from build123d import *

# Parameters (mm, degrees)
F0_W      = 114.494712
F0_H      = 62.637055
F1_DEPTH  = 25.4
F2_R      = 10.795138
F2_R_2    = 10.841205
F2_R_3    = 10.79514
F3_DEPTH  = 116.84
F5_DEPTH  = 42.926
F6_W      = 51.59115
F6_H      = 62.667213
F7_DEPTH  = 11.176
F8_R      = 10.847006
F9_DEPTH  = 65.532
F10_W     = 18.654421
F10_H     = 20.111804
F10_W_2   = 18.65442
F10_H_2   = 17.488524
F11_DEPTH = 45.212


with BuildPart() as f1:
    # F0 (on Front) → F1 (new body)
    with BuildSketch(Plane.XZ):
        with Locations((-4.824847, 5.261216)):
            Rectangle(F0_W, F0_H)
    extrude(amount=F1_DEPTH)

    # F2 (on Front) → F3 (cut)
    with BuildSketch(Plane.XZ):
        with Locations((13.092266, 4.241542)):
            Circle(F2_R)
        with Locations((-28.568659, 5.406883)):
            Circle(F2_R_2)
        with Locations((-28.568659, 5.406883)):
            Circle(F2_R_3, mode=Mode.SUBTRACT)
        with Locations((-28.568659, 5.406883)):
            Circle(F2_R_3)
    extrude(amount=F3_DEPTH, mode=Mode.SUBTRACT)

    # F4 (on Front) → F5 (join)
    with BuildSketch(Plane.XZ):
        Polygon((-42.860791, -25.608312), (-42.860791, 36.285762), (-62.284995, 36.472697), (-62.284995, -26.409047), align=None)
    extrude(amount=F5_DEPTH)

    # F6 (on Front) → F7 (join)
    with BuildSketch(Plane.XZ):
        with Locations((-36.28869, 5.246557)):
            Rectangle(F6_W, F6_H)
    extrude(amount=-F7_DEPTH)

    # F8 (on Front) → F9 (cut)
    with BuildSketch(Plane.XZ):
        with Locations((-26.232786, 2.563626)):
            Circle(F8_R)
    extrude(amount=-F9_DEPTH, mode=Mode.SUBTRACT)

    # F10 (on Front) → F11 (join)
    with BuildSketch(Plane.XZ):
        with Locations((42.555411, -15.739673)):
            Rectangle(F10_W, F10_H)
        with Locations((42.55541, 27.835902)):
            Rectangle(F10_W_2, F10_H_2)
    extrude(amount=F11_DEPTH)


solid = f1.part
The listing builds one solid part. Answer for the finished solid, in the listing's coordinates (mm). A direction names the side the tool comes from. Give positions to 0.01 mm unless a question says otherwise; leave off trailing zeros. Loops run counter-clockwise (first coordinate to the right, second up) from the corner with the lowest first, then second, coordinate; pieces in that order, holes last. Notation, with made-up numbers: (-17, 86) - (22, 86) arc R18 cw to (22, 95) - close; hole circle Ø9 at (72, 12). An arc over 180 degrees is marked (long way). Use one line per item in the form item = value.
1. Section C-C on x = 39 is taken. Give the vertices of the cut face in (y, z).
Calculated:
outline = (-45.21, -25.8) - (-25.4, -25.8) - (-25.4, -26.06) - (0, -26.06) - (0, 36.58) - (-45.21, 36.58) - (-45.21, 19.09) - (-25.4, 19.09) - (-25.4, -5.68) - (-45.21, -5.68) - close
2. Section D-D on x = 17.5 is taken. Give the vertices of the cut face in (y, z), then the cut area to 3 significant figures.
Calculated:
outline = (-25.4, -26.06) - (0, -26.06) - (0, -5.61) - (-25.4, -5.61) - close; (-25.4, 14.1) - (0, 14.1) - (0, 36.58) - (-25.4, 36.58) - close
area = 1,090 mm^2
3. The mould has two halves that part along X. Classify faces 1 (the face through (-10.493, 6, 5)), 2 (the face through (42, -22, 36.58)), 3 (the face through (33.228, -35, -16)): pulls with the +X half, pulls with the -X half, needs draft (parallel to the pull), parting line crosses it, or undercut.
Calculated:
face_1 = pulls with the +X half
face_2 = needs draft
face_3 = undercut
4. Find the intervals of material crossed by line 1 along X through (y, z) = (-39, -6) (3 decimals); line 2 along Z through (x, y) = (35, -40.5); line 3 along Y through (x, z) = (42, -3), in increasing order. Write a range as [from, to].
Calculated:
line_1 = [-62.285, -42.861], [33.228, 51.883]
line_2 = [-25.8, -5.68], [19.09, 36.58]
line_3 = [-25.4, 0]
5. Section B-B on z = 7 is taken. Count the separate pieces of the cut face and the enclosed holes in it, then the cut area to 3 significant figures.
Calculated:
separate_pieces = 3
enclosed_holes = 0
area = 2,530 mm^2
6. Given pin 1 Ø5.5 at (y, z) = (-34, 17.5) entering from +X; pin 2 Ø25 at (x, z) = (13.09, 4.24) entering from -Y; pin 3 Ø10 at (y, z) = (-26, 6) entering from +X; pin 4 Ø21 at (x, z) = (-33, 10.5) entering from -Y, each flat-ended and moving along its own axis, determine where each tip first touches the part or whether it passes through.
Calculated:
pin_1 = 51.88
pin_2 = -25.4
pin_3 = 52.42
pin_4 = -42.93
7. Which of the six approach directions +Z, -Z, +X, -X, +Y, -Y give full straight-line access (tool end or side, diameter ignored) to faces 4 (the face through (-21, 0, -3)), 5 (the face through (42, -35, -5.684)), 6 (the face through (42, -35, -25.796))?
Calculated:
face_4 = +Y
face_5 = +X, -Y
face_6 = -Z, +X, -Y
8. Section A-A on y = -38.5 is taken. Give the vertices of the cut face in (x, z) (3 decimals), then the cut area to 3 significant figures.
Calculated:
outline = (-62.285, -26.409) - (-42.861, -25.608) - (-42.861, 36.286) - (-62.285, 36.473) - close; (33.228, -25.796) - (51.883, -25.796) - (51.883, -5.684) - (33.228, -5.684) - close; (33.228, 19.092) - (51.883, 19.092) - (51.883, 36.58) - (33.228, 36.58) - close
area = 1,910 mm^2
